Design review of the part shown in the three views and the two pictorial views. Dimensions are in mm from the part's minimum x, y and z. A direction names the side the tool comes from. Give positions to 0.01 mm unless a question says otherwise; leave off trailing zeros. Loops run counter-clockwise (first coordinate to the right, second up) from the corner with the lowest first, then second, coordinate; pieces in that order, holes last. Notation, with made-up numbers: (51.5, 13) -> (108.5, 13) arc R21 cw to (108.5, 27) -> close; hole circle Ø10 at (-27.75, 15). An arc over 180 degrees is marked (long way). Answer as CSV lines item,"result". Start each with the question number.
Item 1: For L1, parallel to Y at x = 9.5, z = 0.5; L2, parallel to Z at x = 2, y = 5; L3, parallel to Z at x = 12.25, y = 6.5, list the stretches that pass through material, from the lowest coordinate up. Write a range as from..to.
Item 2: Add section A-A on z = 0.5. State the section outline as (x, y) points (1 decimal).
Item 3: Add section C-C on x = 2.75. State the section outline as (y, z) points, plus the area to 3 significant figures.
Item 4: Machinability: for the marked faces 1 and 2, which of the approach directions +Z, -Z, +X, -X, +Y, -Y give a long, thin tool a straight path to every point of the face, cutting with its end or side? Answer none if there is none.
Item 5: The part is to be moulded in two halves that separate along Y. For the marked faces 3, 4 and 5, say which applies: +Y half, -Y half, draft (parallel to the pull), parting line (faces both ways), or undercut.
Item 6: Clearance check with flat-ended pins moving along their axes: P1, Ø3, axis at x = 12, y = 5.5, coming from the -Z side; P2, Ø2, axis at x = 14.5, z = 6, coming from the -Y side (1 decimal); P3, Ø6, axis at x = 8, y = 10.5, coming from the +Z side; P4, Ø5, axis at x = 9, y = 11, coming from the -Z side. State where each tip first meets the part, or that it passes through.
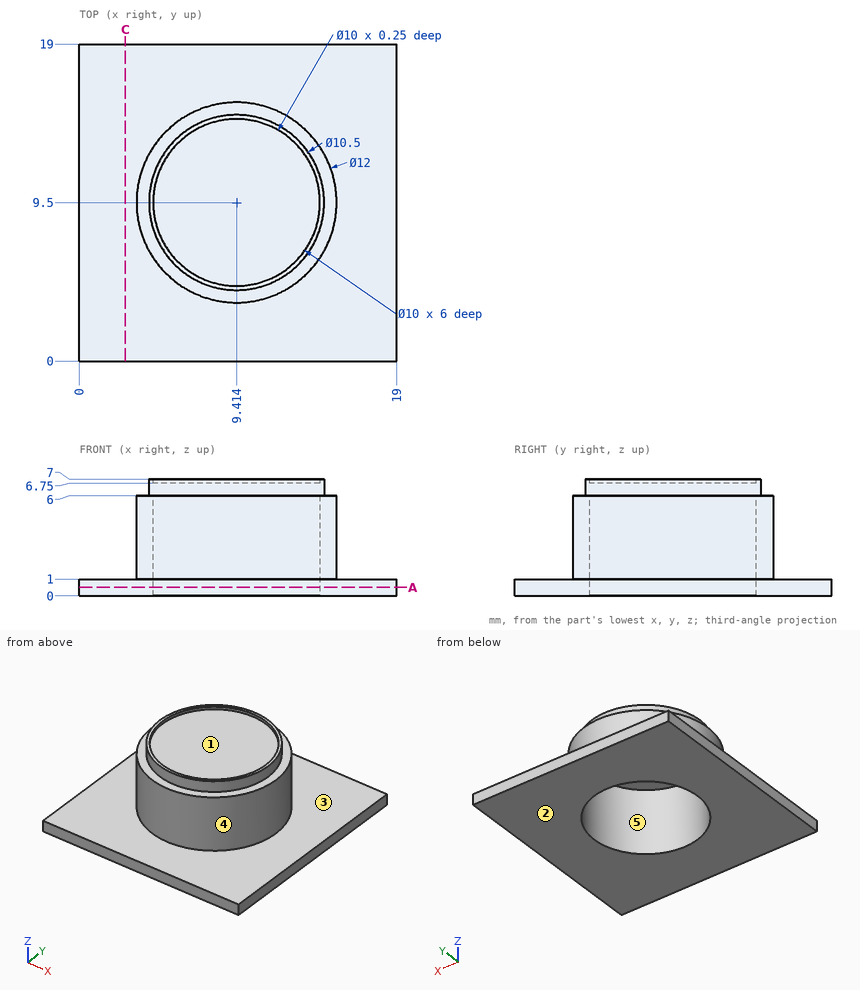
Computed values:
1,L1,"0..4.5, 14.5..19"
1,L2,"0..1"
1,L3,"6..6.75"
2,outline,"(0, 0) -> (19, 0) -> (19, 19) -> (0, 19) -> close; hole circle Ø10 at (9.4, 9.5)"
3,outline,"(0, 0) -> (19, 0) -> (19, 1) -> (0, 1) -> close"
3,area,"19.0 mm²"
4,face 1,"+Z"
4,face 2,"-Z, +X, -X, +Y, -Y"
5,face 3,"draft"
5,face 4,"parting line"
5,face 5,"undercut"
6,P1,"z = 0"
6,P2,"y = 5.1"
6,P3,"z = 6.75"
6,P4,"z = 6"
